```python
from build123d import *


with BuildPart() as part:
    # Sketch1 → Revolve1 (revolve)
    with BuildSketch(Plane(origin=(0, 0, 0), x_dir=(1, 0, 0), z_dir=(0, 1, 0))):
        with BuildLine():
            Line((-35, 0), (-35, 8.528910447))
            ThreePointArc((-35, 8.528910447), (-35.148501992, 9.461090209), (-35.579306073, 10.300982937))
            Line((-35.579306073, 10.300982937), (-48.702751771, 28.22792751))
            ThreePointArc((-48.702751771, 28.22792751), (-49.282057844, 30), (-48.702751771, 31.77207249))
            Line((-48.702751771, 31.77207249), (-35.579306073, 49.699017063))
            ThreePointArc((-35.579306073, 49.699017063), (-35.148501992, 50.538909791), (-35, 51.471089553))
            Line((-35, 51.471089553), (-35, 60))
            Line((-35, 60), (-33.5, 60))
            Line((-33.5, 60), (-33.5, 50.980726369))
            ThreePointArc((-33.5, 50.980726369), (-33.648501992, 50.048546606), (-34.079306073, 49.208653878))
            Line((-34.079306073, 49.208653878), (-46.843780693, 31.77207249))
            ThreePointArc((-46.843780693, 31.77207249), (-47.423086766, 30), (-46.843780693, 28.22792751))
            Line((-46.843780693, 28.22792751), (-34.079306073, 10.791346122))
            ThreePointArc((-34.079306073, 10.791346122), (-33.648501992, 9.951453394), (-33.5, 9.019273631))
            Line((-33.5, 9.019273631), (-33.5, 0))
            Line((-33.5, 0), (-35, 0))
        make_face()
    revolve(axis=Axis((0, 0, -72.546995865), (0, 0, 1)))


solid = part.part
```
Geometry: final body of the model. Coordinates: model frame, mm. A direction names the side the tool comes from. Round coordinates to 2 decimals unless told otherwise and drop trailing zeros. Loops run counter-clockwise (first coordinate to the right, second up) from the corner with the lowest first, then second, coordinate; pieces in that order, holes last. Notation, with made-up numbers: (71, 62) -> (120, 62) arc R16 cw to (120, 69) -> close; hole circle Ø7 at (86, 62.25). An arc over 180 degrees is marked (long way). Write each question's results on one line, items separated by ' | '.
Item 1: Line query: probe 1 along X at (y, z) = (0, -54.5); probe 2 along X at (y, z) = (-15.5, -9). Output: solid intervals per line, ascending. Write a range as [from, to].
Answers below:
probe 1: x = [-35, -33.5], [33.5, 35] | probe 2: x = [-31.42, -29.7], [29.7, 31.42]
Item 2: Set-up query: faces 1 (the face through (7.561, 34.048, -48.118)), 2 (the face through (7.851, 35.355, -48.829)), 3 (the face through (28, 21, -4)). Return all of +Z, -Z, +X, -X, +Y, -Y with unobstructed straight access to the full face (end or side cutting, diameter ignored); none if empty.
Answers below:
face 1: none | face 2: -Z | face 3: +Z
Item 3: Pull-direction query (Z, two-part tool) for faces 4 (the face through (28, 21, -56)), 5 (the face through (0, 34, 0)), 6 (the face through (27.54, 21.11, -11.64)); classes: pulls with the +Z half, pulls with the -Z half, needs draft (parallel to the pull), parting line crosses it, or undercut.
Answers below:
face 4: needs draft | face 5: pulls with the +Z half | face 6: undercut
Item 4: Cut plane C-C on z = -42.5. Return the cut outline in (x, y).
Answers below:
outline: circle Ø81.7 at (0, 0); hole circle Ø77.98 at (0, 0)
Item 5: Pin query (flat end, axial travel): pin 1 Ø2 at (x, z) = (-35.5, -20.5) entering from -Y; pin 2 Ø8 at (y, z) = (3, -9.5) entering from -X; pin 3 Ø2 at (x, z) = (-26, -40) entering from -Y. Return the tip coordinate at first contact, or that it passes through.
Answers below:
pin 1: stops at y = -26.22 | pin 2: stops at x = -37.82 | pin 3: stops at y = -35.03
Item 6: Cut plane D-D on z = -24.5. Return the cut outline in (x, y), and give its area (3 significant figures).
Answers below:
outline: circle Ø91.95 at (0, 0); hole circle Ø88.23 at (0, 0) | area: 526 mm²
